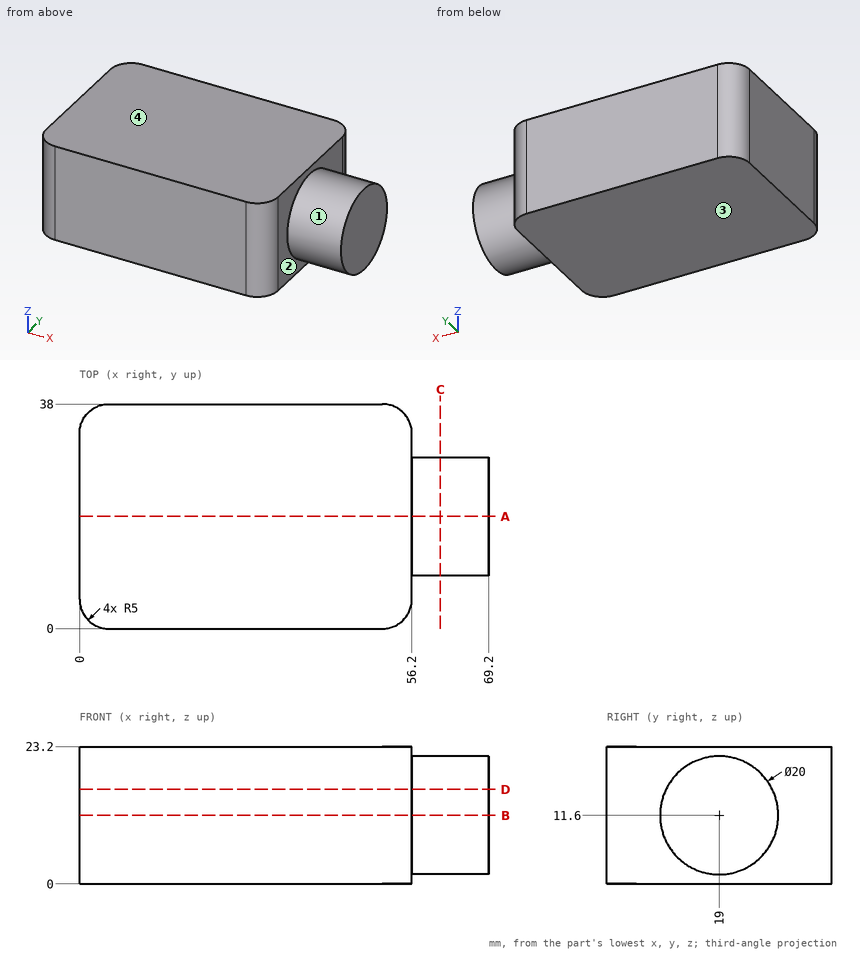
Part print with two shaded views. Sizes in mm from the minimum x, y, z corner. Coordinates: 2 decimals unless noted, no trailing zeros. Write each loop counter-clockwise with the first axis right and the second up, starting at its lowest first coordinate (ties: lowest second). Pieces come first, ordered by that corner, then holes.
1. Band-saw the part on D-D, the plane z = 16. Give the cut face in (x, y), and give its area (3 significant figures).
Answer block:
outline: (0, 5) arc R5 ccw to (5, 0) - (51.2, 0) arc R5 ccw to (56.2, 5) - (56.2, 10.02) - (69.2, 10.02) - (69.2, 27.98) - (56.2, 27.98) - (56.2, 33) arc R5 ccw to (51.2, 38) - (5, 38) arc R5 ccw to (0, 33) - close
area: 2,350 mm2
2. Band-saw the part on C-C, the plane x = 61. Give the cut face in (y, z), and give its area (3 significant figures).
Answer block:
outline: circle Ø20 at (19, 11.6)
area: 314 mm2
3. Pull direction Z, two halves, no side cores. Call the marked faces 1, 2, 3 and 4: released by +Z, released by -Z, zero draft, split by the parting line, or undercut.
Answer block:
face 1: split by the parting line
face 2: zero draft
face 3: released by -Z
face 4: released by +Z
4. Drill centre lines: probe 1 along X at (y, z) = (28.5, 7); probe 2 along Y at (x, z) = (60, 20.75); probe 3 along Y at (x, z) = (64, 8.75). Where is each one in solid material? Low to high.
Answer block:
probe 1: x = 0 to 56.2
probe 2: y = 14.97 to 23.03
probe 3: y = 9.41 to 28.59
5. Drop flat-ended pins along their axis: pin 1 (4 mm diameter, centred on x = 61, z = 7.5, fed in from +Y); pin 2 (1 mm diameter, centred on x = 9.5, y = 9, fed in from -Z); pin 3 (8 mm diameter, centred on x = 56, z = 3.5, fed in from -Y); pin 4 (3 mm diameter, centred on x = 56, z = 17.5, fed in from +Y). Give the stop position or say it passes through.
Answer block:
pin 1: stops at y = 28.78
pin 2: stops at z = 0
pin 3: stops at y = 0.06
pin 4: stops at y = 36.76
6. Band-saw the part on A-A, the plane y = 19. Give the cut face in (x, z), and give its area (3 significant figures).
Answer block:
outline: (0, 0) - (56.2, 0) - (56.2, 1.6) - (69.2, 1.6) - (69.2, 21.6) - (56.2, 21.6) - (56.2, 23.2) - (0, 23.2) - close
area: 1,560 mm2
7. Band-saw the part on B-B, the plane z = 11.6. Give the cut face in (x, y), and give its area (3 significant figures).
Answer block:
outline: (0, 5) arc R5 ccw to (5, 0) - (51.2, 0) arc R5 ccw to (56.2, 5) - (56.2, 9) - (69.2, 9) - (69.2, 29) - (56.2, 29) - (56.2, 33) arc R5 ccw to (51.2, 38) - (5, 38) arc R5 ccw to (0, 33) - close
area: 2,370 mm2
